Build history of the part. All positions in model axes, mm. A direction names the side the tool comes from. Give positions to 0.01 mm unless a question says otherwise; leave off trailing zeros. Write each loop counter-clockwise with the first axis right and the second up, starting at its lowest first coordinate (ties: lowest second). Pieces come first, ordered by that corner, then holes.
Autodesk Inventor part; units mm, degrees
ref_plane "YZ Plane" through (0, 0, 0) normal (1, 0, 0) x (0, 1, 0)
ref_plane "XZ Plane" through (0, 0, 0) normal (0, 1, 0) x (-1, 0, 0)
ref_plane "XY Plane" through (0, 0, 0) normal (0, 0, 1) x (1, 0, 0)
sketch "Boceto1" plane through (0, 0, 0) normal (0, 0, 1) x (1, 0, 0)
  line L0 (17.3205, 30) -> (34.641, 0)
  line L1 (34.641, 0) -> (17.3205, -30)
  line L2 (17.3205, -30) -> (-17.3205, -30)
  line L3 (-17.3205, -30) -> (-34.641, 0)
  line L4 (-34.641, 0) -> (-17.3205, 30)
  line L5 (-17.3205, 30) -> (17.3205, 30)
  point P0 (0, 0)
  point P1 (0, 0)
  dimension "d0" = 30
extrude "Extrusión1" add sketch "Boceto1" along normal blind 5
sketch "Boceto3" plane through (0, 0, 5) normal (0, 0, 1) x (1, 0, 0)
  circle A0 centre (0, 0) radius 9
  dimension "d5" = 18
extrude "Extrusión3" cut sketch "Boceto3" against normal blind 10
sketch "Boceto4" plane through (0, 0, 5) normal (0, 0, 1) x (1, 0, 0)
  circle A0 centre (0, 0) radius 9
  line L0 (-6.15, 6.571) -> (6.15, 6.571)
  line L1 (6.15, 6.571) -> (6.15, -17.029)
  line L2 (6.15, -17.029) -> (-6.15, -17.029)
  line L3 (-6.15, -17.029) -> (-6.15, 6.571)
  point P0 (0, 6.571)
  dimension "d10" = 12.3
  dimension "d11" = 23.6
extrude "Extrusión4" cut sketch "Boceto4" against normal blind 3 contours L1 A0 L3 L0 | L1 L2 L3 A0
sketch "Boceto5" plane through (0, 0, 5) normal (0, 0, 1) x (1, 0, 0)
  line L0 (6.15, -17.029) -> (-6.15, -17.029)
  line L1 (34.641, 0) -> (17.3205, 30)
  line L2 (-34.641, 0) -> (-17.3205, -30)
  line L3 (-17.3205, -30) -> (17.3205, -30)
  line L4 (17.3205, -30) -> (34.641, 0)
  line L5 (6.5197, 15.6925) -> (11.6697, 24.6126)
  line L6 (11.6697, 24.6126) -> (15.4803, 22.4126)
  line L7 (15.4803, 22.4126) -> (10.3303, 13.4925)
  line L8 (10.3303, 13.4925) -> (6.5197, 15.6925)
  line L9 (6.5197, 15.6925) -> (15.4803, 22.4126) construction
  line L10 (11.6697, 24.6126) -> (10.3303, 13.4925) construction
  line L11 (-16.85, -2.2) -> (-27.15, -2.2)
  line L12 (-27.15, -2.2) -> (-27.15, 2.2)
  line L13 (-27.15, 2.2) -> (-16.85, 2.2)
  line L14 (-16.85, 2.2) -> (-16.85, -2.2)
  line L15 (-16.85, -2.2) -> (-27.15, 2.2) construction
  line L16 (-27.15, -2.2) -> (-16.85, 2.2) construction
  line L17 (6.5197, -15.6925) -> (11.6697, -24.6126)
  line L18 (11.6697, -24.6126) -> (15.4803, -22.4126)
  line L19 (15.4803, -22.4126) -> (10.3303, -13.4925)
  line L20 (10.3303, -13.4925) -> (6.5197, -15.6925)
  line L21 (6.5197, -15.6925) -> (15.4803, -22.4126) construction
  line L22 (11.6697, -24.6126) -> (10.3303, -13.4925) construction
  arc A0 (6.15, -6.571) -> (-6.15, -6.571) centre (0, 0) ccw
  line L23 (-17.3205, 30) -> (-34.641, 0)
  line L24 (0, 0) -> (17.3205, 30)
  line L25 (0, 0) -> (17.3205, -30)
  line L26 (-27.15, -2.2) -> (-22.85, -2.2)
  line L27 (-27.15, -2.2) -> (-22.75, -2.2)
  line L28 (-22.75, -2.2) -> (-22.75, -6.6)
  line L29 (-22.75, -6.6) -> (-27.15, -6.6)
  line L30 (-27.15, -6.6) -> (-27.15, -2.2)
  line L31 (15.4803, -22.4126) -> (13.2803, -18.6021)
  line L32 (13.2803, -18.6021) -> (17.0908, -16.4021)
  line L33 (17.0908, -16.4021) -> (19.2908, -20.2126)
  line L34 (19.2908, -20.2126) -> (15.4803, -22.4126)
  line L35 (11.6697, 24.6126) -> (9.4697, 20.8021)
  line L36 (9.4697, 20.8021) -> (5.6592, 23.0021)
  line L37 (5.6592, 23.0021) -> (7.8592, 26.8126)
  line L38 (7.8592, 26.8126) -> (11.6697, 24.6126)
  line L39 (15.4803, 22.4126) -> (19.2908, 20.2126)
  line L40 (19.2908, 20.2126) -> (17.4071, 16.95)
  line L41 (17.4071, 16.95) -> (13.5966, 19.15)
  line L42 (13.5966, 19.15) -> (15.4803, 22.4126)
  line L43 (11.6697, -24.6126) -> (8.0324, -26.7126)
  line L44 (8.0324, -26.7126) -> (5.8324, -22.9021)
  line L45 (5.8324, -22.9021) -> (9.4697, -20.8021)
  line L46 (9.4697, -20.8021) -> (11.6697, -24.6126)
  line L47 (-27.15, 2.2) -> (-27.15, 6.5)
  line L48 (-27.15, 6.5) -> (-22.85, 6.5)
  line L49 (-22.85, 6.5) -> (-22.85, 2.2)
  line L50 (-22.85, 2.2) -> (-27.15, 2.2)
  point P0 (11, 19.0526)
  point P1 (-22, 0)
  point P2 (11, -19.0526)
  point P3 (-22, 0)
  point P4 (-22, 0)
  point P5 (12.5, 21.6506)
  point P6 (13.575, 23.5126)
  point P7 (11, 19.0526)
  point P8 (11, -19.0526)
  point P9 (12.5, -21.6506)
  point P10 (-27.15, 0)
  point P11 (13.575, -23.5126)
  dimension "d16" = 4.4
  dimension "d17" = 10.3
  dimension "d18" = 4.4
  dimension "d20" = 4.4
  dimension "d21" = 10.3
  dimension "d47" = 22
  dimension "d48" = 22
  dimension "d49" = 22
  dimension "d60" = 4.4
  dimension "d61" = 4.4
  dimension "d62" = 4.4
  dimension "d63" = 4.4
  dimension "d64" = 4.4
  dimension "d65" = 4.4
  dimension "d68" = 4.4
  dimension "d69" = 4.4
  dimension "d70" = 4.3
sketch "Boceto9" plane through (0, 0, 0) normal (0, 0, -1) x (-1, 0, 0)
  circle A0 centre (0, 0) radius 9
  circle A1 centre (0, 0) radius 12
  circle A2 centre (0, 0) radius 9
extrude "Extrusión9" add sketch "Boceto9" along normal blind 3
extrude "Extrusión11" cut sketch "Boceto5" against normal blind 10 contours L24 L8 L5 L6 | L6 L7 L8 L24 | L25 L20 L19 L18 | L18 L17 L20 L25 | L5 L36 L37 L38 | L39 L40 L41 L7 | L43 L44 L45 L17 | L19 L32 L33 L34 | L11 L12 L13 L14 | L28 L29 L30 L11 | L13 L47 L48 L49
properties part number "Base"
1. Mould opens along X. For faces 5 (the face through (25.86, 15.21, 2.46)), 6 (the face through (7.974, 18.212, 2.535)), 7 (the face through (0, 30, 2)), 8 (the face through (-22.85, 4, 3)) say: pulls with the +X half, pulls with the -X half, needs draft (parallel to the pull), parting line crosses it, or undercut.
2. 3-axis set-ups, long thin cutter, end or side, ignore diameter. For faces 1 (the face through (11.99, -0.53, -1.48)), 2 (the face through (6.948, -24.834, 2.535)), 3 (the face through (0, -13, 2)), 4 (the face through (0, -30, 2)): which of +Z, -Z, +X, -X, +Y, -Y reach the whole face in a straight line?
3. Saw through at C-C on z = -1.25. Give the cut face in (x, y), plus the area to 3 significant figures.
4. Drill centre lines: line 1 along X through (y, z) = (0, 1.45); line 2 along Y through (x, z) = (12, 1.25); line 3 along Y through (x, z) = (0, 2.9). Where is each one in solid material? Low to high.
5. Saw through at B-B on y = 3. Give the cut face in (x, z).
6. Drop flat-ended pins along their axis: pin 1 (1.5 mm diameter, centred on x = -20, z = 2, fed in from +Y); pin 2 (20.5 mm diameter, centred on x = 0, y = 0, fed in from +Z); pin 3 (1 mm diameter, centred on x = 0, y = -15.5, fed in from -Z); pin 4 (3.5 mm diameter, centred on y = 4, z = 1.5, fed in from -X). Give the stop position or say it passes through.
7. Saw through at A-A on x = 0. Give the cut face in (y, z).
8. Saw through at D-D on x = -19. Give the cut face in (y, z).
Outcome:
1. face 5: pulls with the +X half
1. face 6: undercut
1. face 7: needs draft
1. face 8: undercut
2. face 1: -Z
2. face 2: +Z, -Z
2. face 3: +Z
2. face 4: +Z, -Z, +X, -X, -Y
3. outline: circle Ø24 at (0, 0); hole circle Ø18 at (0, 0)
3. area: 198 mm2
4. line 1: x = -34.64 to -27.15, -16.85 to -9, 9 to 34.64
4. line 2: y = -30 to -24.42, -16.38 to 16.38, 24.42 to 30
4. line 3: y = -30 to -17.03, 9 to 30
5. outline: (-32.91, 0) - (-27.15, 0) - (-27.15, 5) - (-32.91, 5) - close; (-22.85, 0) - (-11.62, 0) - (-11.62, -3) - (-8.49, -3) - (-8.49, 5) - (-22.85, 5) - close; (8.49, -3) - (11.62, -3) - (11.62, 0) - (32.91, 0) - (32.91, 5) - (8.49, 5) - close
6. pin 1: stops at y = 26.66
6. pin 2: stops at z = 5
6. pin 3: stops at z = 0
6. pin 4: stops at x = -33.34
7. outline: (-30, 0) - (-12, 0) - (-12, -3) - (-9, -3) - (-9, 2) - (-17.03, 2) - (-17.03, 5) - (-30, 5) - close; (9, -3) - (12, -3) - (12, 0) - (30, 0) - (30, 5) - (9, 5) - close
8. outline: (-27.09, 0) - (-2.2, 0) - (-2.2, 5) - (-27.09, 5) - close; (2.2, 0) - (27.09, 0) - (27.09, 5) - (2.2, 5) - close
